```python
from build123d import *

# Parameters (mm, degrees)
F0_W     = 10
F0_H     = 500
F1_DEPTH = 500
F3_DEPTH = 10
F5_DEPTH = 10
F6_W     = 10
F6_H     = 10
F7_DEPTH = 1


with BuildPart() as f1:
    # F0 (on Top) → F1 (new body)
    with BuildSketch(Plane.XY):
        with Locations((-12.096023, 214.334732)):
            Rectangle(F0_W, F0_H)
    extrude(amount=F1_DEPTH)

    # F2 (on face) → F3 (cut)
    with BuildSketch(Plane(origin=(-17.096023, 0, 0), x_dir=(0, -1, 0), z_dir=(-1, 0, 0))):
        Polygon((35.665268, 500), (-464.334732, 500), (35.665268, 0), align=None)
    extrude(amount=-F3_DEPTH, mode=Mode.SUBTRACT)

    # F4 (on face) → F5 (cut)
    with BuildSketch(Plane.YZ.offset(-7.096023)):
        Polygon((461.334732, 493.5), (-25.665268, 6.5), (461.334732, 6.5), align=None)
    extrude(amount=-F5_DEPTH, mode=Mode.SUBTRACT)

    # F6 (on face) → F7 (join)
    with BuildSketch(Plane(origin=(0, 464.334732, 0), x_dir=(-1, 0, 0), z_dir=(0, 1, 0))):
        with Locations((12.096023, 495)):
            Rectangle(F6_W, F6_H)
    extrude(amount=F7_DEPTH)


solid = f1.part
```
The model under review builds one solid part; all positions refer to its coordinate system, in mm. Round coordinates to 2 decimals unless told otherwise and drop trailing zeros. Write each loop counter-clockwise with the first axis right and the second up, starting at its lowest first coordinate (ties: lowest second). Pieces come first, ordered by that corner, then holes. Notation, with made-up numbers: (14.25, 73) - (19.25, 73) arc R24 cw to (19.25, 85) - close; hole circle Ø6 at (-37.5, 66). An arc over 180 degrees is marked (long way). Use one line per item in the form item = value.
Q1. Consider section B-B (x = -12). State the section outline as (y, z) points, and give its area (3 significant figures).
Answer key:
outline = (-35.67, 0) - (464.33, 0) - (464.33, 490) - (465.33, 490) - (465.33, 500) - (464.33, 500) - close; hole (-25.67, 6.5) - (461.33, 6.5) - (461.33, 493.5) - close
area = 6,430 mm2
Q2. Consider section C-C (z = 424.5). State the section outline as (x, y) points, and give its area (3 significant figures).
Answer key:
outline = (-17.1, 388.83) - (-7.1, 388.83) - (-7.1, 392.33) - (-17.1, 392.33) - close; (-17.1, 461.33) - (-7.1, 461.33) - (-7.1, 464.33) - (-17.1, 464.33) - close
area = 65.0 mm2
Q3. Insertion check: pin 1 Ø2 at (x, z) = (-15, 385) entering from -Y; pin 2 Ø3 at (x, z) = (-12.5, 322.5) entering from +Y. Each pin has a flat end and moves straight along its axis. Give the tip position at first contact, or say it passes through.
Answer key:
pin_1 = 348.33
pin_2 = 464.33
Q4. For line 1 (Z direction, x = -11.5, y = 145.5); line 2 (Z direction, x = -14.25, y = 350); line 3 (Y direction, x = -16.25, z = 143.5), list the stretches that pass through material, from the lowest coordinate up. Write a range as [from, to].
Answer key:
line_1 = [0, 6.5], [177.67, 181.17]
line_2 = [0, 6.5], [382.17, 385.67]
line_3 = [107.83, 111.33], [461.33, 464.33]
Q5. Consider section A-A (y = 292). State the section outline as (x, z) points, and give its area (3 significant figures).
Answer key:
outline = (-17.1, 0) - (-7.1, 0) - (-7.1, 6.5) - (-17.1, 6.5) - close; (-17.1, 324.17) - (-7.1, 324.17) - (-7.1, 327.67) - (-17.1, 327.67) - close
area = 100 mm2
Q6. Draft analysis for pull direction Z (two halves, no side actions). For faces 1 (the flat face through (-12.026, 221.244, 253.409)), 2 (the flat face through (-12.166, 217.835, 253.5)), 3 (the flat face through (-17.096, 214, 249)), state which applies: +Z half, -Z half, draft (parallel to the pull), parting line (faces both ways), or undercut.
Answer key:
face_1 = undercut
face_2 = +Z half
face_3 = draft
